Could you check a few things on this drawing? It's one solid part, dimensions in mm from its lowest x, y, z. A direction names the side the tool comes from. Give positions to 0.01 mm unless a question says otherwise; leave off trailing zeros. Loops run counter-clockwise (first coordinate to the right, second up) from the corner with the lowest first, then second, coordinate; pieces in that order, holes last. Notation, with made-up numbers: (-20.5, 51.5) - (0.5, 51.5) arc R33 ccw to (0.5, 85.5) - close; hole circle Ø11 at (-6.5, 80.25). An arc over 180 degrees is marked (long way). Answer as a JSON object with one key per item and string values.
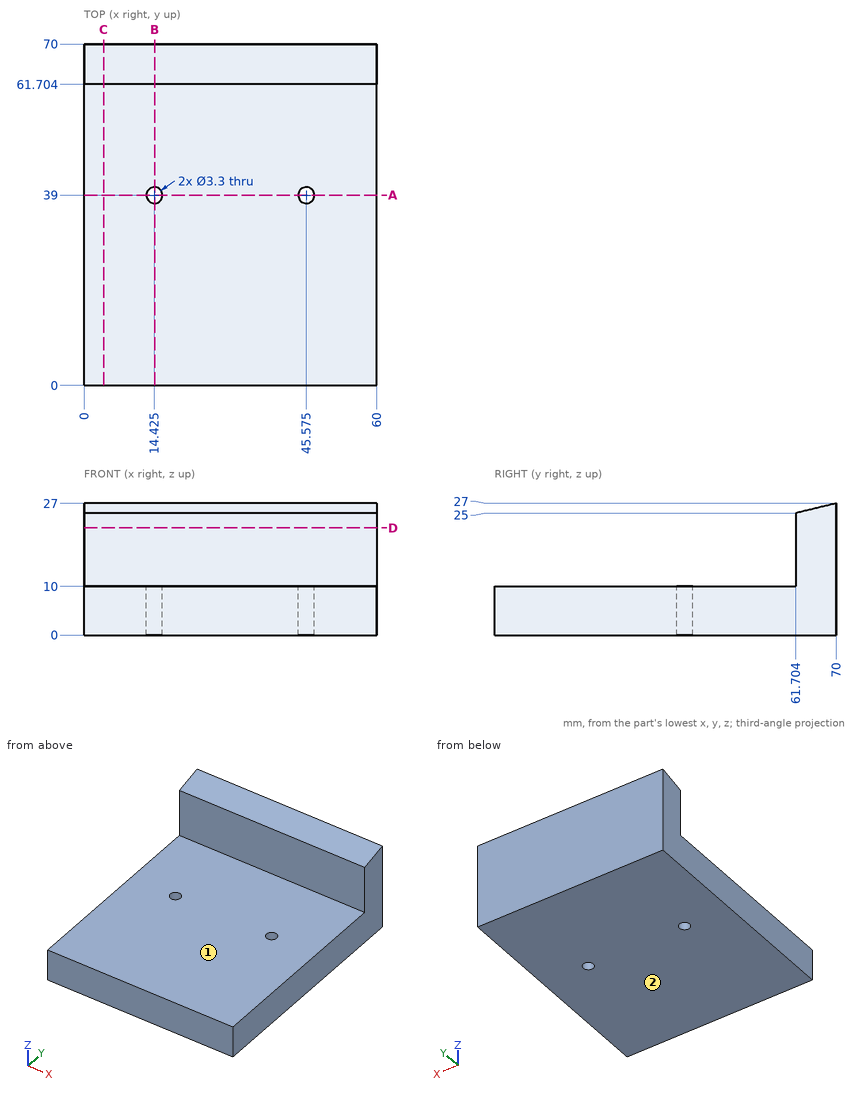
1) I'm going to push a flat-ended pin straight in: P1, Ø1, axis at x = 38.5, y = 55, coming from the +Z side. Where does the tip first touch, or does it pass through?
Check sheet entries:
{"P1": "z = 10"}
2) Imagine slicing it at C-C on x = 4. Write out the boundary of the cut face in (y, z).
Check sheet entries:
{"outline": "(0, 0) - (70, 0) - (70, 27) - (61.7, 25) - (61.7, 10) - (0, 10) - close"}
3) Imagine slicing it at D-D on z = 22. Write out the boundary of the cut face in (x, y).
Check sheet entries:
{"outline": "(0, 61.7) - (60, 61.7) - (60, 70) - (0, 70) - close"}
4) Which directions (+Z, -Z, +X, -X, +Y, -Y) give clear straight access to the entire face, cutting with the end or side of a thin tool? Please do the marked faces 1 and 2.
Check sheet entries:
{"face 1": "+Z, +X, -X, -Y", "face 2": "-Z, +X, -X, +Y, -Y"}
5) Imagine slicing it at B-B on x = 14.5. Write out the boundary of the cut face in (y, z).
Check sheet entries:
{"outline": "(0, 0) - (37.35, 0) - (37.35, 10) - (0, 10) - close; (40.65, 0) - (70, 0) - (70, 27) - (61.7, 25) - (61.7, 10) - (40.65, 10) - close"}
6) Imagine slicing it at A-A on y = 39. Write out the boundary of the cut face in (x, z) (3 decimals).
Check sheet entries:
{"outline": "(0, 0) - (12.775, 0) - (12.775, 10) - (0, 10) - close; (16.075, 0) - (43.925, 0) - (43.925, 10) - (16.075, 10) - close; (47.225, 0) - (60, 0) - (60, 10) - (47.225, 10) - close"}
7) I need wall thicknesses on L1, parallel to X at y = 38, z = 5.25; L2, parallel to Y at x = 10, z = 23.5; L3, parallel to Z at x = 25, y = 4.5. Which ranges of each line are inside material? Lowest first, please.
Check sheet entries:
{"L1": "0 to 13.11, 15.74 to 44.26, 46.89 to 60", "L2": "61.7 to 70", "L3": "0 to 10"}
